Could you check a few things on this drawing? It's one solid part, dimensions in mm from its lowest x, y, z. A direction names the side the tool comes from. Give positions to 0.01 mm unless a question says otherwise; leave off trailing zeros. Write each loop counter-clockwise with the first axis right and the second up, starting at its lowest first coordinate (ties: lowest second). Pieces come first, ordered by that corner, then holes. Notation, with made-up numbers: M -5,-34 L 52,-34 A13 cw 52,-27 Z; hole C 61.25,83.25 d1. An arc over 180 degrees is marked long. Answer as CSV lines item,"result". Start each with the question number.
Q1. On a 3-axis mill with a long thin cutter (end or side, diameter ignored), from which of +Z, -Z, +X, -X, +Y, -Y can I reach the whole of each face in a straight line? I mean the marked faces 4 and 5. Say none if no direction works.
Q2. Suppose I cut it at B-B (z = 4.5). Write out the boundary of the cut face in (x, y), then the cut area to 3 significant figures.
Q3. For pin 1 (1 mm diameter, centred on y = 2, z = 5, fed in from -X), with a flat end and sliding along its axis, tell me the tip position at first contact or that it passes through.
Q4. Suppose I cut it at C-C (z = 6.25). Write out the boundary of the cut face in (x, y).
Q5. Thinking about a two-plate mould opening in Z: for the marked faces 1, 2 and 3, which applies, +Z half, -Z half, draft (parallel to the pull), parting line (faces both ways), or undercut?
Q6. Suppose I cut it at A-A (x = 4.5). Write out the boundary of the cut face in (y, z), then the cut area to 3 significant figures.
Q7. If I drill on line 1 along Z through (x, y) = (4.5, 2.3); line 2 along Z through (x, y) = (3.5, 0.55); line 3 along Y through (x, z) = (3, 0.5), over which ranges is the centre line in solid material (lowest first)?
Q8. Suppose I cut it at D-D (y = 1). Write out the boundary of the cut face in (x, z).
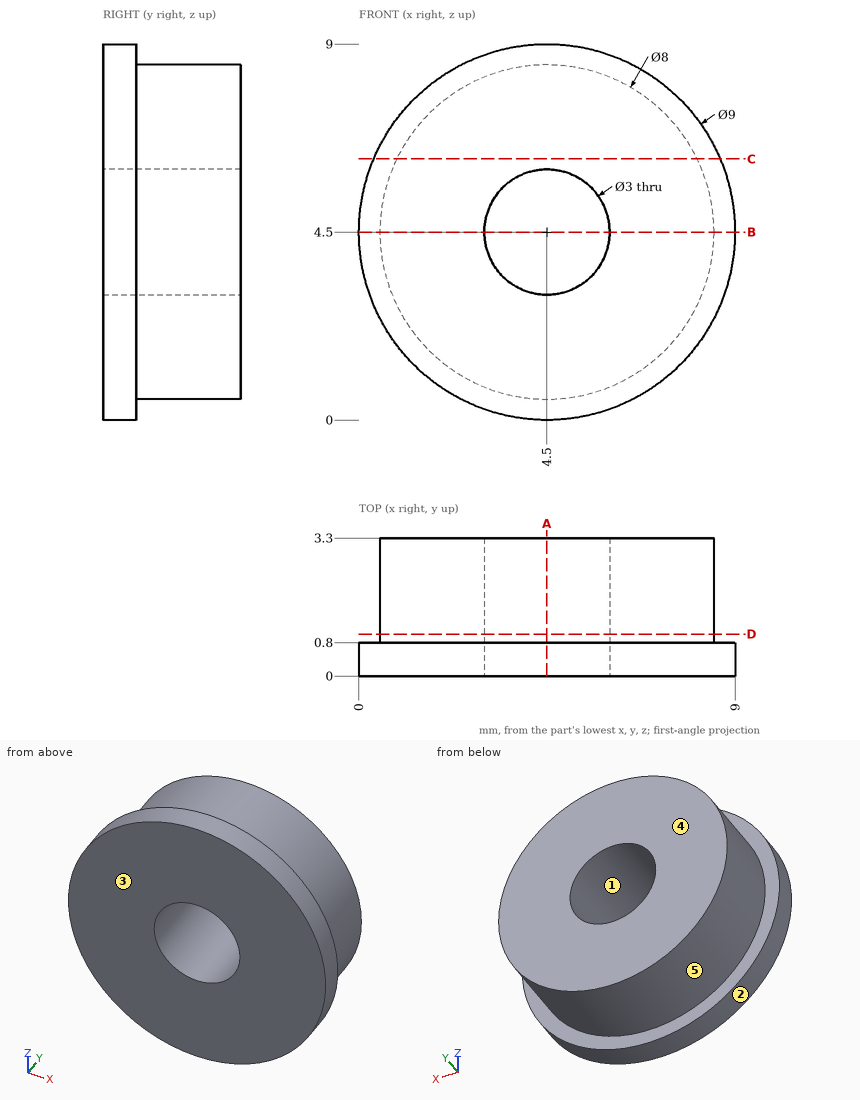
Resolved:
1,face 4,"+Z, -Z, +X, -X, +Y"
1,face 5,"+Y"
2,outline,"M 0,0 L 3,0 L 3,3.3 L 0.5,3.3 L 0.5,0.8 L 0,0.8 Z; M 6,0 L 9,0 L 9,0.8 L 8.5,0.8 L 8.5,3.3 L 6,3.3 Z"
2,area,"17.3 mm^2"
3,pin 1,"x = 0.5"
4,outline,"M 0.35,0 L 8.65,0 L 8.65,0.8 L 8.1,0.8 L 8.1,3.3 L 0.9,3.3 L 0.9,0.8 L 0.35,0.8 Z"
5,face 1,"undercut"
5,face 2,"parting line"
5,face 3,"draft"
6,outline,"M 0,0 L 0.8,0 L 0.8,0.5 L 3.3,0.5 L 3.3,3 L 0,3 Z; M 0,6 L 3.3,6 L 3.3,8.5 L 0.8,8.5 L 0.8,9 L 0,9 Z"
6,area,"17.3 mm^2"
7,line 1,"0.5 to 3, 6 to 8.5"
7,line 2,"0.11 to 3.38, 5.62 to 8.89"
7,line 3,"0 to 0.8"
8,outline,"C 4.5,4.5 d8; hole C 4.5,4.5 d3"
